```python
from build123d import *

# Parameters (mm, degrees)
BOSS_EXTRUDE1_DEPTH      = 6.35
BOSS_EXTRUDE1_DEPTH_BACK = 6.35
SKETCH3_R                = 4.7625
SKETCH3_R_2              = 2.7686
CHAMFER1_SIZE            = 0.19939


with BuildPart() as part:
    # Sketch3 → Boss-Extrude1 (new, two sides: drawn at the far end of the back side and taken through both)
    with BuildSketch(Plane.XY.offset(-BOSS_EXTRUDE1_DEPTH_BACK)):
        Circle(SKETCH3_R)
        Circle(SKETCH3_R_2, mode=Mode.SUBTRACT)
    extrude(amount=BOSS_EXTRUDE1_DEPTH + BOSS_EXTRUDE1_DEPTH_BACK)

    # Chamfer1
    chamfer1_edges = [part.edges().sort_by_distance(p)[0] for p in [
        (-4.7625, 0, -6.35),
        (-2.7686, 0, -6.35),
        (-4.7625, 0, 6.35),
        (-2.7686, 0, 6.35),
    ]]
    chamfer(chamfer1_edges, length=CHAMFER1_SIZE)


solid = part.part
```
Read the model definition and answer for the solid it produces. Units are mm, in the model's axes. Coordinates: 2 decimals unless noted, no trailing zeros. Write each loop counter-clockwise with the first axis right and the second up, starting at its lowest first coordinate (ties: lowest second). Pieces come first, ordered by that corner, then holes. Notation, with made-up numbers: (62.5, -1.75) - (72.5, -1.75) arc R20 ccw to (72.5, 10.25) - close; hole circle Ø3 at (-4, 2). An arc over 180 degrees is marked (long way). Answer as a JSON object with one key per item and string values. Group by question number.
1. Each of these flat-tipped pins is pushed along its axis until it touches: P1, Ø2, axis at y = -2.5, z = 1, coming from the +X side; P2, Ø5, axis at y = -3.5, z = -1.5, coming from the +X side; P3, Ø1, axis at y = -2.5, z = 3, coming from the -X side. Where does it stop, or does it pass through?
2. A cutting plane is placed at A-A (y = 0). Determine the outline of the cut face in (x, z).
3. Consider L1, parallel to Y at x = 0, z = -3.5; L2, parallel to X at y = 1.75, z = -3; L3, parallel to X at y = -0.75, z = -1.75. Determine where each line is inside the solid, lowest interval first. Write a range as [from, to].
4. The mould has two halves that part along Y. Classify faces 1 (the cylindrical face through (-2.2, -1.68, -0.09)), 2 (the flat face through (3, -1, 6.35)), 3 (the cylindrical face through (-3.78, -2.9, -0.09)): +Y half, -Y half, draft (parallel to the pull), parting line (faces both ways), or undercut.
5. A cutting plane is placed at C-C (z = 2.25). Determine the outline of the cut face in (x, y) (1 decimal).
Worked out:
{
 "1": {"P1": "stops at x = 4.52", "P2": "stops at x = 4.66", "P3": "stops at x = -4.32"},
 "2": {"outline": "(-4.76, -6.15) - (-4.56, -6.35) - (-2.97, -6.35) - (-2.77, -6.15) - (-2.77, 6.15) - (-2.97, 6.35) - (-4.56, 6.35) - (-4.76, 6.15) - close; (2.77, -6.15) - (2.97, -6.35) - (4.56, -6.35) - (4.76, -6.15) - (4.76, 6.15) - (4.56, 6.35) - (2.97, 6.35) - (2.77, 6.15) - close"},
 "3": {"L1": "y = [-4.76, -2.77], [2.77, 4.76]", "L2": "x = [-4.43, -2.15], [2.15, 4.43]", "L3": "x = [-4.7, -2.67], [2.67, 4.7]"},
 "4": {"face 1": "undercut", "face 2": "draft", "face 3": "parting line"},
 "5": {"outline": "circle Ø9.5 at (0, 0); hole circle Ø5.5 at (0, 0)"}
}
